Model file for the job. Use its own axes, mm. Give positions to 0.01 mm unless a question says otherwise; leave off trailing zeros. Write each loop counter-clockwise with the first axis right and the second up, starting at its lowest first coordinate (ties: lowest second). Pieces come first, ordered by that corner, then holes. Notation, with made-up numbers: (-31.5, -7.75) - (-12.5, -7.75) arc R9 cw to (-12.5, 0.25) - close; hole circle Ø6 at (78.25, 1.25). An arc over 180 degrees is marked (long way). Use a Markdown table: item, result. Add a question column.
```python
from build123d import *

# Parameters (mm, degrees)
SKETCH2_R               = 12.5
SKETCH2_R_2             = 2.65
BOSS_EXTRUDE2_DEPTH     = 0.8
FILLET1_R               = 1
CUT_EXTRUDE1_DEPTH      = 238.711107019
CUT_EXTRUDE1_DEPTH_BACK = 238.711107019
SKETCH5_R               = 1.725
FILLET2_R               = 0.5


with BuildPart() as part:
    # Sketch2 → Boss-Extrude2 (new body)
    with BuildSketch(Plane.XY):
        with BuildLine():
            Line((1, -171.98), (3.883580208, -171.98))
            ThreePointArc((3.883580208, -171.98), (4.7625, -166.83), (5.641419792, -171.98))
            Line((5.641419792, -171.98), (30.871080208, -171.98))
            ThreePointArc((30.871080208, -171.98), (31.75, -166.83), (32.628919792, -171.98))
            Line((32.628919792, -171.98), (56.271080208, -171.98))
            ThreePointArc((56.271080208, -171.98), (57.15, -166.83), (58.028919792, -171.98))
            Line((58.028919792, -171.98), (81.671080208, -171.98))
            ThreePointArc((81.671080208, -171.98), (82.55, -166.83), (83.428919792, -171.98))
            Line((83.428919792, -171.98), (107.071080208, -171.98))
            ThreePointArc((107.071080208, -171.98), (107.95, -166.83), (108.828919792, -171.98))
            Line((108.828919792, -171.98), (132.471080208, -171.98))
            ThreePointArc((132.471080208, -171.98), (133.35, -166.83), (134.228919792, -171.98))
            Line((134.228919792, -171.98), (159.458580208, -171.98))
            ThreePointArc((159.458580208, -171.98), (160.3375, -166.83), (161.216419792, -171.98))
            Line((161.216419792, -171.98), (164.1, -171.98))
            Line((164.1, -171.98), (164.1, 0))
            Line((164.1, 0), (1, 0))
            Line((1, 0), (1, -171.98))
        make_face()
        with Locations((82.55, -85)):
            Circle(SKETCH2_R, mode=Mode.SUBTRACT)
        with Locations((69.85, -3.175)):
            Circle(SKETCH2_R_2, mode=Mode.SUBTRACT)
        with Locations((6.35, -94.25)):
            Circle(SKETCH2_R_2, mode=Mode.SUBTRACT)
        with Locations((6.35, -68.85)):
            Circle(SKETCH2_R_2, mode=Mode.SUBTRACT)
        with Locations((6.35, -43.45)):
            Circle(SKETCH2_R_2, mode=Mode.SUBTRACT)
        with Locations((6.35, -18.05)):
            Circle(SKETCH2_R_2, mode=Mode.SUBTRACT)
        with Locations((19.05, -3.175)):
            Circle(SKETCH2_R_2, mode=Mode.SUBTRACT)
        with Locations((44.45, -3.175)):
            Circle(SKETCH2_R_2, mode=Mode.SUBTRACT)
        with Locations((146.05, -3.175)):
            Circle(SKETCH2_R_2, mode=Mode.SUBTRACT)
        with Locations((158.75, -18.05)):
            Circle(SKETCH2_R_2, mode=Mode.SUBTRACT)
        with Locations((158.75, -43.45)):
            Circle(SKETCH2_R_2, mode=Mode.SUBTRACT)
        with Locations((158.75, -94.25)):
            Circle(SKETCH2_R_2, mode=Mode.SUBTRACT)
        with Locations((158.75, -68.85)):
            Circle(SKETCH2_R_2, mode=Mode.SUBTRACT)
        with Locations((95.25, -3.175)):
            Circle(SKETCH2_R_2, mode=Mode.SUBTRACT)
        with Locations((120.65, -3.175)):
            Circle(SKETCH2_R_2, mode=Mode.SUBTRACT)
    extrude(amount=BOSS_EXTRUDE2_DEPTH)

    # Fillet1
    fillet1_edges = [part.edges().sort_by_distance(p)[0] for p in [
        (1, -171.98, 0.4),
        (1, 0, 0.4),
        (164.1, 0, 0.4),
        (164.1, -171.98, 0.4),
    ]]
    fillet(fillet1_edges, radius=FILLET1_R)

    # Sketch5 → Cut-Extrude1 (cut, two sides: drawn at the far end of the back side and taken through both)
    with BuildSketch(Plane.XY.offset(0.8).offset(-CUT_EXTRUDE1_DEPTH_BACK)):
        with Locations((42.775, -43.995)):
            Circle(SKETCH5_R)
        with Locations((122.325, -43.995)):
            Circle(SKETCH5_R)
        with Locations((122.325, -115.985)):
            Circle(SKETCH5_R)
        with Locations((42.775, -115.985)):
            Circle(SKETCH5_R)
    extrude(amount=CUT_EXTRUDE1_DEPTH + CUT_EXTRUDE1_DEPTH_BACK, mode=Mode.SUBTRACT)

    # Fillet2
    fillet2_edges = [part.edges().sort_by_distance(p)[0] for p in [
        (81.671080208, -171.98, 0.4),
        (58.028919792, -171.98, 0.4),
        (56.271080208, -171.98, 0.4),
        (32.628919792, -171.98, 0.4),
        (30.871080208, -171.98, 0.4),
        (5.641419792, -171.98, 0.4),
        (3.883580208, -171.98, 0.4),
        (161.216419792, -171.98, 0.4),
        (159.458580208, -171.98, 0.4),
        (134.228919792, -171.98, 0.4),
        (132.471080208, -171.98, 0.4),
        (108.828919792, -171.98, 0.4),
        (107.071080208, -171.98, 0.4),
        (83.428919792, -171.98, 0.4),
    ]]
    fillet(fillet2_edges, radius=FILLET2_R)


solid = part.part
```
(1) Band-saw the part on A-A (x = 19.05). Write the cut outline in (y, z) (3 decimals), then the cut area to 3 significant figures.
(2) Flat gauge pins, fed straight in: pin 1 (6 mm diameter, centred on x = 57.15, y = -169.48, fed in from -Z); pin 2 (5 mm diameter, centred on x = 19.05, y = -3.175, fed in from +Z). Where does each tip first touch, or does it go through?
(3) Band-saw the part on D-D (z = 0.55). Give the number of separate pieces and of enclosed holes in the cut face, then the cut area to 3 significant figures.
(4) Band-saw the part on B-B (y = -68.85). Write the cut outline in (x, z), then the cut area to 3 significant figures.
(5) Band-saw the part on C-C (y = -94.25). Write the cut outline in (x, z).
(6) Two-plate mould, pull along Y, no slides. Class faces 1 (the cylindrical face through (5.78, -20.64, 0.39)), 2 (the flat face through (100, -85, 0.8)): +Y half, -Y half, draft (parallel to the pull), parting line (faces both ways), or undercut.
(7) Probe probe 1 along Y at (x, z) = (107.95, 0.6); probe 2 along X at (y, z) = (-88, 0.7); probe 3 along Y at (x, z) = (158.75, 0.3). List the from-to ranges inside material, lowest first. Write a range as [from, to].
Model answer:
| question | item | result |
|---|---|---|
| 1 | outline | (-171.98, 0) - (-5.825, 0) - (-5.825, 0.8) - (-171.98, 0.8) - close; (-0.525, 0) - (0, 0) - (0, 0.8) - (-0.525, 0.8) - close |
| 1 | area | 133 mm^2 |
| 2 | pin 1 | stops at z = 0 |
| 2 | pin 2 | passes through |
| 3 | separate pieces | 1 |
| 3 | enclosed holes | 19 |
| 3 | area | 27,100 mm^2 |
| 4 | outline | (1, 0) - (3.7, 0) - (3.7, 0.8) - (1, 0.8) - close; (9, 0) - (156.1, 0) - (156.1, 0.8) - (9, 0.8) - close; (161.4, 0) - (164.1, 0) - (164.1, 0.8) - (161.4, 0.8) - close |
| 4 | area | 122 mm^2 |
| 5 | outline | (1, 0) - (3.7, 0) - (3.7, 0.8) - (1, 0.8) - close; (9, 0) - (74.14, 0) - (74.14, 0.8) - (9, 0.8) - close; (90.96, 0) - (156.1, 0) - (156.1, 0.8) - (90.96, 0.8) - close; (161.4, 0) - (164.1, 0) - (164.1, 0.8) - (161.4, 0.8) - close |
| 6 | face 1 | undercut |
| 6 | face 2 | draft |
| 7 | probe 1 | y = [-166.83, 0] |
| 7 | probe 2 | x = [1, 70.42], [94.68, 164.1] |
| 7 | probe 3 | y = [-167.36, -96.9], [-91.6, -71.5], [-66.2, -46.1], [-40.8, -20.7], [-15.4, 0] |
